Autodesk Inventor part; units mm, degrees
ref_plane "YZ Plane" through (0, 0, 0) normal (1, 0, 0) x (0, 1, 0)
ref_plane "XZ Plane" through (0, 0, 0) normal (0, 1, 0) x (-1, 0, 0)
ref_plane "XY Plane" through (0, 0, 0) normal (0, 0, 1) x (1, 0, 0)
sketch "スケッチ1" plane through (0, 0, 0) normal (1, 0, 0) x (0, 1, 0)
  line L0 (125.6523, 179.1954) -> (-64.3477, 179.1954)
  line L1 (-64.3477, 179.1954) -> (-64.3477, -110.8046)
  line L2 (-64.3477, -110.8046) -> (125.6523, -110.8046)
  line L3 (125.6523, -110.8046) -> (125.6523, 179.1954)
  point P0 (0, 0)
  dimension "d0" = 190
  dimension "d1" = 290
extrude "押し出し1" add sketch "スケッチ1" along normal blind 2.6
sketch "スケッチ2" plane through (2.6, 0, 0) normal (1, 0, 0) x (0, 0, -1)
  line L0 (-179.1954, 125.6523) -> (-179.1954, -64.3477)
  line L1 (-179.1954, -64.3477) -> (110.8046, -64.3477)
  line L2 (110.8046, -64.3477) -> (110.8046, 125.6523)
  line L3 (110.8046, 125.6523) -> (-179.1954, 125.6523)
  line L4 (-34.1954, 30.6523) -> (-34.1954, 125.6523)
  line L5 (110.8046, 125.6523) -> (-179.1954, 125.6523)
  line L6 (-34.1954, 30.6523) -> (110.8046, 30.6523)
  point P0 (0, 0)
  point P1 (-169.1954, 115.6523)
  point P2 (100.8046, 115.6523)
  point P3 (-169.1954, -54.3477)
  point P4 (100.8046, -54.3477)
  dimension "d4" = 10
  dimension "d5" = 10
hole "穴1" at (2.6, 115.6523, 169.1954) at (2.6, 115.6523, -100.8046) at (2.6, -54.3477, 169.1954) at (2.6, -54.3477, -100.8046) direction (-1, 0, 0) diameter 4.5 depth 10 tip angle 118
sketch "スケッチ4" plane through (0, 0, 0) normal (-1, 0, 0) x (0, 0, 1)
  line L0 (-73.8046, -49.3477) -> (-73.8046, 109.6523)
  line L1 (-73.8046, 109.6523) -> (136.1954, 109.6523)
  line L2 (136.1954, 109.6523) -> (136.1954, -49.3477)
  line L3 (136.1954, -49.3477) -> (-73.8046, -49.3477)
  point P0 (0, 0)
extrude "押し出し3" cut sketch "スケッチ4" against normal blind 10
sketch "スケッチ5" plane through (0, 0, 0) normal (-1, 0, 0) x (0, 0, 1)
  circle A0 centre (146.6954, 30.1523) radius 5.5
  line L0 (136.1954, 109.6523) -> (136.1954, -49.3477)
  line L1 (136.1954, 38.6523) -> (154.6954, 38.6523)
  line L2 (154.6954, 38.6523) -> (154.6954, 21.6523)
  line L3 (154.6954, 21.6523) -> (136.1954, 21.6523)
  line L4 (136.1954, 21.6523) -> (136.1954, 38.6523)
  point P0 (0, 0)
  point P1 (136.1954, 21.6523)
  dimension "d21" = 8
  dimension "d22" = 8.5
  dimension "d23" = 8.5
extrude "押し出し4" cut sketch "スケッチ5" against normal blind 10 contours A0 | L1 L2 L3 L0
fillet "フィレット1" radius 8 4 edges at (1.3, 38.6523, 154.6954) (1.3, 21.6523, 154.6954) (1.3, 38.6523, 136.1954) (1.3, 21.6523, 136.1954)
properties part number "lc_box_side" material "ポリカーボネート、クリア"
Check sheet for the modelled part. Datum: model origin and axes. Units: mm. A direction names the side the tool comes from. Coordinates: 2 decimals unless noted, no trailing zeros. Write each loop counter-clockwise with the first axis right and the second up, starting at its lowest first coordinate (ties: lowest second). Pieces come first, ordered by that corner, then holes.
Item 1: Cross-section at C-C on x = 0.45. Record the boundary of the cut face in (y, z), then the cut area to 3 significant figures.
Numbers:
outline: (-64.35, -110.8) - (125.65, -110.8) - (125.65, 179.2) - (-64.35, 179.2) - close; hole circle Ø4.5 at (-54.35, -100.8); hole circle Ø4.5 at (-54.35, 169.2); hole (-49.35, -73.8) - (109.65, -73.8) - (109.65, 136.2) - (46.65, 136.2) arc R8 cw to (38.65, 144.2) - (38.65, 146.7) arc R8 ccw to (30.65, 154.7) - (29.65, 154.7) arc R8 ccw to (21.65, 146.7) - (21.65, 144.2) arc R8 cw to (13.65, 136.2) - (-49.35, 136.2) - close; hole circle Ø4.5 at (115.65, -100.8); hole circle Ø4.5 at (115.65, 169.2)
area: 21,300 mm2
Item 2: Cross-section at A-A on z = -59.5. Record the boundary of the cut face in (x, y), then the cut area to 3 significant figures.
Numbers:
outline: (0, -64.35) - (2.6, -64.35) - (2.6, -49.35) - (0, -49.35) - close; (0, 109.65) - (2.6, 109.65) - (2.6, 125.65) - (0, 125.65) - close
area: 80.6 mm2
Item 3: Cross-section at B-B on y = -36.5. Record the boundary of the cut face in (x, z).
Numbers:
outline: (0, -110.8) - (2.6, -110.8) - (2.6, -73.8) - (0, -73.8) - close; (0, 136.2) - (2.6, 136.2) - (2.6, 179.2) - (0, 179.2) - close
Item 4: Access from +Z, -Z, +X, -X, +Y, -Y to the whole of each face (thin tool, end or side, straight path). Record for faces 3 (the face through (1.318, 40.934, 138.601)), 4 (the face through (2.6, -55, 36)).
Numbers:
face 3: +X, -X
face 4: +Z, -Z, +X, +Y, -Y
Item 5: Scan lines: probe 1 along Y at (x, z) = (1.5, -32.5); probe 2 along Z at (x, y) = (2.3, -16); probe 3 along Z at (x, y) = (1.25, -55.5). Record each from-to range of solid material in increasing order.
Numbers:
probe 1: y = -64.35 to -49.35, 109.65 to 125.65
probe 2: z = -110.8 to -73.8, 136.2 to 179.2
probe 3: z = -110.8 to -102.74, -98.87 to 167.26, 171.13 to 179.2
Item 6: Mould release check, pull along Z, two halves, no side actions. Record for faces 1 (the face through (1.32, 36.37, 152.29)), 2 (the face through (0, -55, 36)): released by +Z, released by -Z, zero draft, split by the parting line, or undercut.
Numbers:
face 1: undercut
face 2: zero draft
